Build history of the part. All positions in model axes, mm. Give positions to 0.01 mm unless a question says otherwise; leave off trailing zeros. Loops run counter-clockwise (first coordinate to the right, second up) from the corner with the lowest first, then second, coordinate; pieces in that order, holes last.
1) Band-saw the part on A-A on x = 0. List the corners of the cut face in (y, z), then the cut area to 3 significant figures.
2) Band-saw the part on B-B on y = 0. List the corners of the cut face in (x, z).
3) Band-saw the part on C-C on z = 16. List the corners of the cut face in (x, y).
4) Flat gauge pins, fed straight in: P1, Ø10, axis at y = 20, z = 32.5, coming from the -X side; P2, Ø2, axis at y = 5, z = 38, coming from the -X side; P3, Ø1, axis at y = 14, z = 15.5, coming from the +X side. Where does each tip first touch, or does it go through?
5) Two-plate mould, pull along X, no slides. Class faces 1 (the cylindrical face through (-4.336, -19.524, 24.65)), 2 (the flat face through (-44, 0, 20)), 3 (the cylindrical face through (-65, 0, 10)): +X half, -X half, draft (parallel to the pull), parting line (faces both ways), or undercut.
6) Band-saw the part on D-D on y = 18. List the corners of the cut face in (x, z), then the cut area to 3 significant figures.
7) Wall check: line 1 (Y direction, x = 0, z = 33); line 2 (X direction, y = 0.5, z = 8.5); line 3 (X direction, y = -9, z = 30.5). Give the ranges that are in metal, low to high.
```python
from build123d import *

# Parameters (mm, degrees)
SKETCH1_R           = 20
BOSS_EXTRUDE1_DEPTH = 20
SKETCH2_R           = 30
SKETCH2_R_2         = 20
BOSS_EXTRUDE2_DEPTH = 30


with BuildPart() as part:
    # Sketch1 → Boss-Extrude1 (new body)
    with BuildSketch(Plane.XY):
        with BuildLine():
            Line((-9, 28.618176043), (-54.5, 14.309088021))
            ThreePointArc((-54.5, 14.309088021), (-65, 0), (-54.5, -14.309088021))
            Line((-54.5, -14.309088021), (-9, -28.618176043))
            ThreePointArc((-9, -28.618176043), (0, -30), (9, -28.618176043))
            Line((9, -28.618176043), (54.5, -14.309088021))
            ThreePointArc((54.5, -14.309088021), (65, 0), (54.5, 14.309088021))
            Line((54.5, 14.309088021), (9, 28.618176043))
            ThreePointArc((9, 28.618176043), (0, 30), (-9, 28.618176043))
        make_face()
        Circle(SKETCH1_R, mode=Mode.SUBTRACT)
    extrude(amount=BOSS_EXTRUDE1_DEPTH)

    # Sketch2 → Boss-Extrude2 (add)
    with BuildSketch(Plane.XY.offset(20)):
        with Locations(Location((0, 0, 0), (0, 0, 107.457603124))):
            Circle(SKETCH2_R)
        Circle(SKETCH2_R_2, mode=Mode.SUBTRACT)
    extrude(amount=BOSS_EXTRUDE2_DEPTH)


solid = part.part
```
Findings below:
1. outline: (-30, 0) - (-20, 0) - (-20, 50) - (-30, 50) - close; (20, 0) - (30, 0) - (30, 50) - (20, 50) - close
1. area: 1,000 mm2
2. outline: (-65, 0) - (-20, 0) - (-20, 50) - (-30, 50) - (-30, 20) - (-65, 20) - close; (20, 0) - (65, 0) - (65, 20) - (30, 20) - (30, 50) - (20, 50) - close
3. outline: (-54.5, -14.31) - (-9, -28.62) arc R30 ccw to (9, -28.62) - (54.5, -14.31) arc R15 ccw to (54.5, 14.31) - (9, 28.62) arc R30 ccw to (-9, 28.62) - (-54.5, 14.31) arc R15 ccw to start; hole circle Ø40 at (0, 0)
4. P1: stops at x = -25.98
4. P2: stops at x = -29.73
4. P3: stops at x = 56.54
5. face 1: undercut
5. face 2: draft
5. face 3: -X half
6. outline: (-42.76, 0) - (-8.72, 0) - (-8.72, 50) - (-24, 50) - (-24, 20) - (-42.76, 20) - close; (8.72, 0) - (42.76, 0) - (42.76, 20) - (24, 20) - (24, 50) - (8.72, 50) - close
6. area: 2,280 mm2
7. line 1: y = -30 to -20, 20 to 30
7. line 2: x = -64.99 to -19.99, 19.99 to 64.99
7. line 3: x = -28.62 to -17.86, 17.86 to 28.62
